Geometry: final body of the model. Coordinates: model frame, mm. A direction names the side the tool comes from. Give positions to 0.01 mm unless a question says otherwise; leave off trailing zeros. Loops run counter-clockwise (first coordinate to the right, second up) from the corner with the lowest first, then second, coordinate; pieces in that order, holes last. Notation, with made-up numbers: M 32,50 L 55,50 A13 ccw 55,73 Z; hole C 46,62 d2. An arc over 180 degrees is marked long. Put each result on its own line as item: value.
```python
from build123d import *

# Parameters (mm, degrees)
CROQUIS2_W              = 45
CROQUIS2_H              = 20
SALIENTE_EXTRUIR1_DEPTH = 2
CROQUIS3_R              = 1.5
CORTAR_EXTRUIR1_DEPTH   = 3
CROQUIS4_W              = 28
CROQUIS4_H              = 8
CORTAR_EXTRUIR2_DEPTH   = 3


with BuildPart() as part:
    # Croquis2 → Saliente-Extruir1 (new body)
    with BuildSketch(Plane(origin=(0, 0, 0), x_dir=(1, 0, 0), z_dir=(0, 1, 0))):
        Rectangle(CROQUIS2_W, CROQUIS2_H)
    extrude(amount=SALIENTE_EXTRUIR1_DEPTH)

    # Croquis3 → Cortar-Extruir1 (cut, through all)
    with BuildSketch(Plane(origin=(0, 2, 0), x_dir=(1, 0, 0), z_dir=(0, 1, 0))):
        with Locations((-19.5, 7)):
            Circle(CROQUIS3_R)
        with Locations((19.5, 7)):
            Circle(CROQUIS3_R)
        with Locations((-19.5, -7)):
            Circle(CROQUIS3_R)
        with Locations((19.5, -7)):
            Circle(CROQUIS3_R)
    extrude(amount=-CORTAR_EXTRUIR1_DEPTH, mode=Mode.SUBTRACT)

    # Croquis4 → Cortar-Extruir2 (cut, through all)
    with BuildSketch(Plane(origin=(0, 2, 0), x_dir=(1, 0, 0), z_dir=(0, 1, 0))):
        with Locations((4.5, 0)):
            Rectangle(CROQUIS4_W, CROQUIS4_H)
    extrude(amount=-CORTAR_EXTRUIR2_DEPTH, mode=Mode.SUBTRACT)


solid = part.part
```
Item 1: Pin query (flat end, axial travel): pin 1 Ø2.5 at (x, z) = (-19.5, -7) entering from -Y. Return the tip coordinate at first contact, or that it passes through.
Output values:
pin 1: through
Item 2: Section C-C on y = 0.55. Output: boundary loops of the cut face in (x, z).
Output values:
outline: M -22.5,-10 L 22.5,-10 L 22.5,10 L -22.5,10 Z; hole C -19.5,-7 d3; hole C -19.5,7 d3; hole M -9.5,-4 L 18.5,-4 L 18.5,4 L -9.5,4 Z; hole C 19.5,-7 d3; hole C 19.5,7 d3
Item 3: Section B-B on z = 0.5. Output: boundary loops of the cut face in (x, y).
Output values:
outline: M -22.5,0 L -9.5,0 L -9.5,2 L -22.5,2 Z; M 18.5,0 L 22.5,0 L 22.5,2 L 18.5,2 Z
Item 4: Section D-D on x = 9. Output: boundary loops of the cut face in (y, z).
Output values:
outline: M 0,-10 L 2,-10 L 2,-4 L 0,-4 Z; M 0,4 L 2,4 L 2,10 L 0,10 Z
Item 5: Section A-A on x = -19.5. Output: boundary loops of the cut face in (y, z), then the cut area to 3 significant figures.
Output values:
outline: M 0,-10 L 2,-10 L 2,-8.5 L 0,-8.5 Z; M 0,-5.5 L 2,-5.5 L 2,5.5 L 0,5.5 Z; M 0,8.5 L 2,8.5 L 2,10 L 0,10 Z
area: 28.0 mm²
Item 6: Line query: probe 1 along Z at (x, y) = (-19.5, 0.6); probe 2 along X at (y, z) = (1.5, -7); probe 3 along X at (y, z) = (1.35, 3.25). Output: solid intervals per line, ascending. Write a range as [from, to].
Output values:
probe 1: [-10, -8.5], [-5.5, 5.5], [8.5, 10]
probe 2: [-22.5, -21], [-18, 18], [21, 22.5]
probe 3: [-22.5, -9.5], [18.5, 22.5]
Item 7: Set-up query: faces 5 (the flat face through (0, 2, -5)), 6 (the flat face through (4, 1, 4)). Return all of +Z, -Z, +X, -X, +Y, -Y with unobstructed straight access to the full face (end or side cutting, diameter ignored); none if empty.
Output values:
face 5: +Z, -Z, +X, -X, +Y
face 6: +Y, -Y
Item 8: Mould query, pull axis Z, two halves, no side actions, for faces 1 (the cylindrical face through (18, 1, -7)), 2 (the flat face through (0, 1, -10)), 3 (the flat face through (0, 1, 10)), 4 (the flat face through (-22.5, 1, 0)). Classes: pulls with the +Z half, pulls with the -Z half, needs draft (parallel to the pull), parting line crosses it, or undercut.
Output values:
face 1: undercut
face 2: pulls with the -Z half
face 3: pulls with the +Z half
face 4: needs draft
